```python
from build123d import *

# Parameters (mm, degrees)
SKETCH1_R           = 3
BOSS_EXTRUDE1_DEPTH = 3
FILLET1_R           = 3
CUT_EXTRUDE1_REACH  = 98.569
WELD_SKETCH_W       = 6.05
WELD_SKETCH_H       = 3.05
FILLET2_R           = 0.1


with BuildPart() as part:
    # Sketch1 → Boss-Extrude1 (new body)
    with BuildSketch(Plane(origin=(0, 0, 0), x_dir=(1, 0, 0), z_dir=(0, 1, 0))):
        with BuildLine():
            Line((68.999142959, 24.5), (-45.03, 24.5))
            ThreePointArc((-45.03, 24.5), (-59.42765336, 26.658455117), (-64.053442962, 12.85434626))
            Line((-64.053442962, 12.85434626), (-75.682127835, -19.095202846))
            Line((-75.682127835, -19.095202846), (40.839757142, -61.505700619))
            ThreePointArc((40.839757142, -61.505700619), (63.135225428, -21.192802103), (68.999142959, 24.5))
        make_face()
        with BuildLine():
            ThreePointArc((-66.169745277, -17.768626979), (-67.962762758, -13.923488739), (-64.117624541, -12.130471209))
            ThreePointArc((-64.117624541, -12.130471209), (-58.898093563, -13.529040334), (-53.515000008, -14))
            ThreePointArc((-53.515000008, -14), (-50.515, -17.000000016), (-53.51500004, -20))
            ThreePointArc((-53.51500004, -20), (-59.93998258, -19.43788686), (-66.169745277, -17.768626979))
        make_face(mode=Mode.SUBTRACT)
        with Locations(Location((-53.515, 17, 0), (0, 0, 270))):
            Circle(SKETCH1_R, mode=Mode.SUBTRACT)
        with BuildLine():
            ThreePointArc((51.922241647, -14.457733132), (55.352806586, -14.628825828), (56.374201386, -17.908277181))
            ThreePointArc((56.374201386, -17.908277181), (48.64297905, -36.460001059), (37.807738396, -53.387369951))
            ThreePointArc((37.807738396, -53.387369951), (33.600211268, -53.932086993), (33.055494505, -49.724559828))
            ThreePointArc((33.055494505, -49.724559828), (41.773694842, -36.541404897), (48.499417973, -22.238704473))
            ThreePointArc((48.499417973, -22.238704473), (45.1053197, -21.881948257), (44.241223395, -18.580355359))
            ThreePointArc((44.241223395, -18.580355359), (48.93455056, -1.064619844), (50.515, 17))
            ThreePointArc((50.515, 17), (53.515, 20), (56.515, 17))
            ThreePointArc((56.515, 17), (55.360756251, 1.104384228), (51.922241647, -14.457733132))
        make_face(mode=Mode.SUBTRACT)
    extrude(amount=BOSS_EXTRUDE1_DEPTH)

    # Fillet1
    fillet1_edges = [part.edges().sort_by_distance(p)[0] for p in [
        (68.999142959, 1.5, -24.5),
        (40.839757142, 1.5, 61.505700619),
        (-75.682127835, 1.5, 19.095202846),
        (-64.053442962, 1.5, -12.85434626),
        (-45.03, 1.5, -24.5),
    ]]
    fillet(fillet1_edges, radius=FILLET1_R)

    # weld sketch → Cut-Extrude1 (cut, up to next)
    with BuildSketch(Plane(origin=(0, 3, 0), x_dir=(1, 0, 0), z_dir=(0, 1, 0)), mode=Mode.PRIVATE) as cut_extrude1_sk1:
        with Locations((-41.915170648, -7.723381887)):
            Rectangle(WELD_SKETCH_W, WELD_SKETCH_H)
    cut_extrude1_tool1 = extrude(cut_extrude1_sk1.sketch, amount=-CUT_EXTRUDE1_REACH, mode=Mode.PRIVATE) & part.part
    # weld sketch → Cut-Extrude1 (cut, up to next)
    with BuildSketch(Plane(origin=(0, 3, 0), x_dir=(1, 0, 0), z_dir=(0, 1, 0)), mode=Mode.PRIVATE) as cut_extrude1_sk2:
        with Locations((-17.915170648, -7.723381887)):
            Rectangle(WELD_SKETCH_W, WELD_SKETCH_H)
    cut_extrude1_tool2 = extrude(cut_extrude1_sk2.sketch, amount=-CUT_EXTRUDE1_REACH, mode=Mode.PRIVATE) & part.part
    # weld sketch → Cut-Extrude1 (cut, up to next)
    with BuildSketch(Plane(origin=(0, 3, 0), x_dir=(1, 0, 0), z_dir=(0, 1, 0)), mode=Mode.PRIVATE) as cut_extrude1_sk3:
        with Locations((37.084829352, -7.723381887)):
            Rectangle(WELD_SKETCH_W, WELD_SKETCH_H)
    cut_extrude1_tool3 = extrude(cut_extrude1_sk3.sketch, amount=-CUT_EXTRUDE1_REACH, mode=Mode.PRIVATE) & part.part
    # weld sketch → Cut-Extrude1 (cut, up to next)
    with BuildSketch(Plane(origin=(0, 3, 0), x_dir=(1, 0, 0), z_dir=(0, 1, 0)), mode=Mode.PRIVATE) as cut_extrude1_sk4:
        with Locations((13.084829352, -7.723381887)):
            Rectangle(WELD_SKETCH_W, WELD_SKETCH_H)
    cut_extrude1_tool4 = extrude(cut_extrude1_sk4.sketch, amount=-CUT_EXTRUDE1_REACH, mode=Mode.PRIVATE) & part.part
    add(cut_extrude1_tool1.solids().sort_by_distance((-41.915171, 3, 7.723382))[0], mode=Mode.SUBTRACT)
    add(cut_extrude1_tool2.solids().sort_by_distance((-17.915171, 3, 7.723382))[0], mode=Mode.SUBTRACT)
    add(cut_extrude1_tool3.solids().sort_by_distance((37.084829, 3, 7.723382))[0], mode=Mode.SUBTRACT)
    add(cut_extrude1_tool4.solids().sort_by_distance((13.084829, 3, 7.723382))[0], mode=Mode.SUBTRACT)

    # Fillet2
    fillet2_edges = [part.edges().sort_by_distance(p)[0] for p in [
        (-38.890170648, 1.5, 9.248381887),
        (-44.940170648, 1.5, 9.248381887),
        (-44.940170648, 1.5, 6.198381887),
        (-38.890170648, 1.5, 6.198381887),
        (-14.890170648, 1.5, 9.248381887),
        (-20.940170648, 1.5, 9.248381887),
        (-20.940170648, 1.5, 6.198381887),
        (-14.890170648, 1.5, 6.198381887),
        (10.059829352, 1.5, 9.248381887),
        (10.059829352, 1.5, 6.198381887),
        (16.109829352, 1.5, 6.198381887),
        (16.109829352, 1.5, 9.248381887),
        (40.109829352, 1.5, 6.198381887),
        (40.109829352, 1.5, 9.248381887),
        (34.059829352, 1.5, 9.248381887),
        (34.059829352, 1.5, 6.198381887),
    ]]
    fillet(fillet2_edges, radius=FILLET2_R)


solid = part.part
```
Geometry check sheet. Reference: the model listing, model coordinates, mm. A direction names the side the tool comes from. Coordinates: 2 decimals unless noted, no trailing zeros. Write each loop counter-clockwise with the first axis right and the second up, starting at its lowest first coordinate (ties: lowest second). Pieces come first, ordered by that corner, then holes. Notation, with made-up numbers: M 9,-28.5 L 22,-28.5 A10 ccw 22,-9.5 Z; hole C 58,17 d4. An arc over 180 degrees is marked long. Use one line per item in the form item = value. Start each with the question number.
1) Go/stop test with flat-tipped pins: pin 1 Ø1.4 at (y, z) = (1, 8.5) entering from -X; pin 2 Ø0.9 at (x, y) = (12.5, 2) entering from +Z; pin 3 Ø1.5 at (y, z) = (0.5, 20) entering from +X. Record where each tip stops, or that it passes through.
2) Section check A-A on z = -3. Enter the section's corners in (x, y).
3) Thickness scan on probe 1 along Z at (x, y) = (39, 1.8); probe 2 along Z at (x, y) = (38.5, 1.25); probe 3 along Z at (x, y) = (-40, 1.5). Record the ranges inside material, lowest first. Write a range as from..to.
4) Release check for a two-part mould opening along Z. For faces 1 (the flat face through (10.06, 2, 8)), 2 (the flat face through (12, 3, 6)), 3 (the flat face through (-17.794, 1.479, 40.165)) record: pulls with the +Z half, pulls with the -Z half, needs draft (parallel to the pull), parting line crosses it, or undercut.
5) Section check D-D on z = 33. Enter the section's corners in (x, y), and give its area (3 significant figures).
6) Section check C-C on y = 0.5. State how many separate pieces and enclosed holes the cut face has, and give its area (3 significant figures).
7) Set-up check for faces 4 (the cylindrical face through (68.202, 1.521, -23.683)), 5 (the flat face through (37, 2, 6.198)): record each of +Z, -Z, +X, -X, +Y, -Y from which the full face is reachable in a straight line by a thin tool's end or side.
8) Section check B-B on x = 54. Enter the section's corners in (y, z), and give its area (3 significant figures).
Responses:
q1.pin_1 = -72.08
q1.pin_2 = 51.35
q1.pin_3 = 63.75
q2.outline = M -67.64,0 L 49.57,0 L 49.57,3 L -67.64,3 Z; M 55.62,0 L 68.43,0 L 68.43,3 L 55.62,3 Z
q3.probe_1 = -24.5..6.2, 9.25..41.2, 51.81..60.83
q3.probe_2 = -24.5..6.2, 9.25..41.99, 52.48..60.65
q3.probe_3 = -24.5..6.2, 9.25..32.08
q4.face_1 = undercut
q4.face_2 = needs draft
q4.face_3 = pulls with the +Z half
q5.outline = M -37.48,0 L 43.68,0 L 43.68,3 L -37.48,3 Z; M 50.38,0 L 58.58,0 L 58.58,3 L 50.38,3 Z
q5.area = 268 mm2
q6.separate_pieces = 1
q6.enclosed_holes = 7
q6.area = 8,300 mm2
q7.face_4 = -Z, +X, +Y, -Y
q7.face_5 = +Y, -Y
q8.outline = M 0,-24.5 L 3,-24.5 L 3,-19.96 L 0,-19.96 Z; M 0,6.39 L 3,6.39 L 3,14.04 L 0,14.04 Z; M 0,24.65 L 3,24.65 L 3,42.22 L 0,42.22 Z
q8.area = 89.3 mm2
